Could you check a few things on this model? Use its own coordinates, in mm. A direction names the side the tool comes from. Give positions to 0.01 mm unless a question says otherwise; leave off trailing zeros. Loops run counter-clockwise (first coordinate to the right, second up) from the corner with the lowest first, then second, coordinate; pieces in that order, holes last.
1. For faces 1 (the cylindrical face through (-23.5, 7.42, 2.46)), 2 (the flat face through (-22, -2.463, 6)), 3 (the flat face through (-0.272, 19, 2)), 4 (the flat face through (-23, 9, 5)), 5 (the flat face through (-22, 39.484, 2)), which set-ups out of +Z, -Z, +X, -X, +Y, -Y let a thin tool reach every point of the face, with its end or its side?
2. I need wall thicknesses on line 1 along Y through (x, z) = (-22, 1.15); line 2 along Y through (x, z) = (-8, 1.9); line 3 along Y through (x, z) = (-7, 6). Which ranges of each line are inside material? Lowest first, please.
3. For P1, Ø1.5, axis at y = 13, z = 4, coming from the -X side; P2, Ø21, axis at x = -15.5, y = 12.5, coming from the +Z side; P3, Ø2.5, axis at y = 14, z = 2.5, coming from the +X side, each with a flat end and sliding along its axis, tell me the tip position at first contact or that it passes through.
4. Imagine slicing it at C-C (y = 13.5). List the corners of the cut face in (x, z) for me.
5. Imagine slicing it at D-D (x = -43.5). List the corners of the cut face in (y, z) for me.
6. Thinking about a two-plate mould opening in X: for faces 6 (the flat face through (14.728, -7, 5)), 7 (the flat face through (-23, 9, 0)), 8 (the flat face through (-44.272, 19, 2)), 9 (the cylindrical face through (-23.106, 34.47, 2.465)), which applies, +X half, -X half, draft (parallel to the pull), parting line (faces both ways), or undercut?
7. Imagine slicing it at B-B (x = -8). List the corners of the cut face in (y, z) for me.
8. Imagine slicing it at A-A (x = -22). List the corners of the cut face in (y, z) for me, plus the area to 3 significant figures.
Autodesk Inventor part; units mm, degrees
ref_plane "YZ Plane" through (0, 0, 0) normal (1, 0, 0) x (0, 1, 0)
ref_plane "XZ Plane" through (0, 0, 0) normal (0, 1, 0) x (-1, 0, 0)
ref_plane "XY Plane" through (0, 0, 0) normal (0, 0, 1) x (1, 0, 0)
sketch "Skizze1" plane through (0, 0, 0) normal (0, 0, 1) x (1, 0, 0)
  line L0 (-0.2717, 2) -> (-0.2717, -2.4631)
  arc A0 (-2.2717, 0) -> (-0.2717, 2) centre (-2.2717, 2) ccw
  line L1 (-42.2717, 0) -> (-2.2717, 0)
  arc A1 (-44.2717, 2) -> (-42.2717, 0) centre (-42.2717, 2) ccw
  line L2 (-44.2717, 2) -> (-44.2717, -2.4631)
  line L3 (-44.2717, -2.4631) -> (-59.2717, -2.4631)
  line L4 (-59.2717, -10.4631) -> (-59.2717, -2.4631)
  line L5 (-37.1489, -10.4631) -> (-59.2717, -10.4631)
  line L6 (-37.1489, -7.4631) -> (-37.1489, -10.4631)
  line L7 (-26.4444, -7.4631) -> (-37.1489, -7.4631)
  line L8 (-26.4444, -10.4631) -> (-26.4444, -7.4631)
  line L9 (-18.0989, -10.4631) -> (-26.4444, -10.4631)
  line L10 (-18.0989, -7.4631) -> (-18.0989, -10.4631)
  line L11 (-7.3944, -7.4631) -> (-18.0989, -7.4631)
  line L12 (-7.3944, -10.4631) -> (-7.3944, -7.4631)
  line L13 (14.7283, -10.4631) -> (-7.3944, -10.4631)
  line L14 (14.7283, -10.4631) -> (14.7283, -2.4631)
  line L15 (14.7283, -2.4631) -> (-0.2717, -2.4631)
  circle A2 centre (-22, 7.4835) radius 1.5
  circle A3 centre (-36, 21.4835) radius 1.5
  circle A4 centre (-22, 35.4835) radius 1.5
  circle A5 centre (-8, 21.4835) radius 1.5
  circle A6 centre (-22, 21.4835) radius 18
  circle A7 centre (-22, 21.4835) radius 11
  line L16 (-44.2717, -10.4631) -> (-0.2717, -10.4631)
  line L17 (-0.2717, -10.4631) -> (-0.2717, 39.4835)
  line L18 (-0.2717, 39.4835) -> (-44.2717, 39.4835)
  line L19 (-44.2717, 39.4835) -> (-44.2717, -10.4631)
  point P0 (0, 0)
extrude "Extrusion1" add sketch "Skizze1" along normal blind 5 contours L0 L17 L13 L12 L11 L10 L9 L8 L7 L6 L5 L19 L2 A1 L1 A0 | A6 | A0 L1 A1 L19 L18 L17 | L15 L14 L13 L17 | L16 L10 L11 L12 | L19 L5 L4 L3 | L16 L6 L7 L8
sketch "Skizze2" plane through (0, 0, 5) normal (0, 0, 1) x (1, 0, 0)
  line L0 (-59.2717, -10.4631) -> (14.7283, -10.4631)
  line L1 (14.7283, -10.4631) -> (14.7283, -2.4631)
  line L2 (-59.2717, -10.4631) -> (14.7283, -10.4631)
  line L3 (14.7283, -10.4631) -> (14.7283, -2.4631)
  line L4 (14.7283, -2.4631) -> (-59.2717, -2.4631)
  line L5 (-59.2717, -2.4631) -> (-59.2717, -10.4631)
  point P0 (0, 0)
extrude "Extrusion2" add sketch "Skizze2" along normal blind 5
properties part number "Shoulder_stepper_holder" material "ABS-Kunststoff - Schwarz"
Derived:
1. face 1: +Z, -Z
1. face 2: +Z, +Y
1. face 3: +Z, -Z, +X, +Y
1. face 4: +Z, +X, -X, +Y
1. face 5: +Z, -Z, +X, -X, +Y
2. line 1: y = -10.46 to 5.98, 8.98 to 10.48, 32.48 to 33.98, 36.98 to 39.48
2. line 2: y = -10.46 to 19.98, 22.98 to 39.48
2. line 3: y = -10.46 to -2.46
3. P1: stops at x = -44.27
3. P2: stops at z = 5
3. P3: stops at x = -0.27
4. outline: (-44.27, 0) - (-29.57, 0) - (-29.57, 5) - (-44.27, 5) - close; (-14.43, 0) - (-0.27, 0) - (-0.27, 5) - (-14.43, 5) - close
5. outline: (-10.46, 0) - (39.48, 0) - (39.48, 5) - (-2.46, 5) - (-2.46, 10) - (-10.46, 10) - close
6. face 6: +X half
6. face 7: draft
6. face 8: -X half
6. face 9: undercut
7. outline: (-10.46, 0) - (19.98, 0) - (19.98, 5) - (-2.46, 5) - (-2.46, 10) - (-10.46, 10) - close; (22.98, 0) - (39.48, 0) - (39.48, 5) - (22.98, 5) - close
8. outline: (-10.46, 0) - (5.98, 0) - (5.98, 5) - (-2.46, 5) - (-2.46, 10) - (-10.46, 10) - close; (8.98, 0) - (10.48, 0) - (10.48, 5) - (8.98, 5) - close; (32.48, 0) - (33.98, 0) - (33.98, 5) - (32.48, 5) - close; (36.98, 0) - (39.48, 0) - (39.48, 5) - (36.98, 5) - close
8. area: 150 mm2
